CAD build for the part. Positions are in the model's coordinates, mm. Give positions to 0.01 mm unless a question says otherwise; leave off trailing zeros. Order: outer loops, then holes, each group sorted by start corner. A loop starts at its lowest first (then second) coordinate and runs counter-clockwise, first axis right, second up. Notation, with made-up numbers: (21.5, 73.5) -> (42.5, 73.5) arc R22 cw to (42.5, 110.5) -> close; hole circle Ø4 at (-0.75, 80). An arc over 180 degrees is marked (long way). Answer as CSV lines item,"result".
```python
from build123d import *

# Parameters (mm, degrees)
SKETCH_W     = 32
SKETCH_H     = 20.2
PAD_DEPTH    = 1.6
SKETCH003_R  = 0.5
POCKET_DEPTH = 1.601
SKETCH004_W  = 1.6
SKETCH004_H  = 3.1
PAD003_DEPTH = 2.15


with BuildPart() as part:
    # Sketch → Pad (new body)
    with BuildSketch(Plane.XY):
        with Locations((16, 10.1)):
            Rectangle(SKETCH_W, SKETCH_H)
    extrude(amount=PAD_DEPTH)

    # Sketch003 → Pocket (cut, through all)
    with BuildSketch(Plane.XY):
        with Locations((30, 18.939)):
            Circle(SKETCH003_R)
        with Locations((30, 1.563)):
            Circle(SKETCH003_R)
    extrude(amount=POCKET_DEPTH, mode=Mode.SUBTRACT)

    # Sketch004 → Pad003 (join)
    with BuildSketch(Plane.XY):
        with Locations((30.2, 10.1)):
            Rectangle(SKETCH004_W, SKETCH004_H)
    extrude(amount=PAD003_DEPTH)


solid = part.part
```
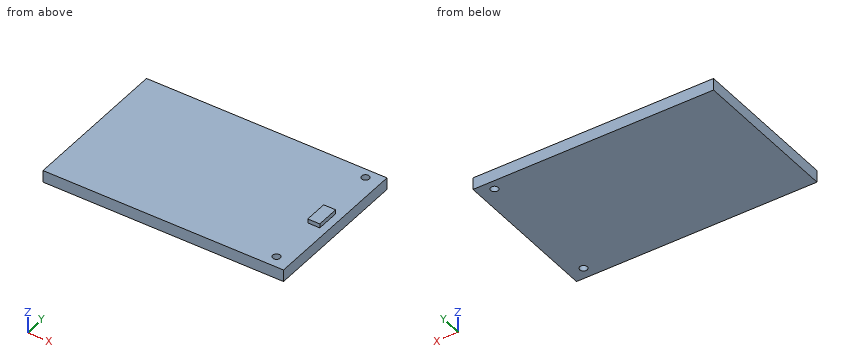
1) Wall check: line 1 along Y through (x, z) = (30, 0.9); line 2 along Z through (x, y) = (26.5, 15.5); line 3 along X through (y, z) = (10, 1.75). Give the ranges that are in metal, low to high. Write a range as [from, to].
Data:
line 1,"y = [0, 1.06], [2.06, 18.44], [19.44, 20.2]"
line 2,"z = [0, 1.6]"
line 3,"x = [29.4, 31]"
2) Pin check, flat tips, straight feed: P1, Ø0.6, axis at x = 30.5, z = 2, coming from the +Y side; P2, Ø1.5, axis at x = 26.5, y = 2.5, coming from the +Z side; P3, Ø0.6, axis at y = 9.5, z = 2, coming from the -X side. Stop position of each tip, or through.
Data:
P1,"stops at y = 11.65"
P2,"stops at z = 1.6"
P3,"stops at x = 29.4"
3) Band-saw the part on C-C, the plane y = 12.5. Write the cut outline in (x, z).
Data:
outline,"(0, 0) -> (32, 0) -> (32, 1.6) -> (0, 1.6) -> close"
4) Band-saw the part on B-B, the plane x = 25. Write the cut outline in (y, z).
Data:
outline,"(0, 0) -> (20.2, 0) -> (20.2, 1.6) -> (0, 1.6) -> close"
5) Band-saw the part on A-A, the plane x = 30. Write the cut outline in (y, z), then the cut area to 3 significant figures.
Data:
outline,"(0, 0) -> (1.06, 0) -> (1.06, 1.6) -> (0, 1.6) -> close; (2.06, 0) -> (18.44, 0) -> (18.44, 1.6) -> (11.65, 1.6) -> (11.65, 2.15) -> (8.55, 2.15) -> (8.55, 1.6) -> (2.06, 1.6) -> close; (19.44, 0) -> (20.2, 0) -> (20.2, 1.6) -> (19.44, 1.6) -> close"
area,"30.8 mm2"
